from build123d import *

# Parameters (mm, degrees)
SKETCH1_W           = 69.85
SKETCH1_H           = 25.4
SKETCH1_R           = 6.35
BOSS_EXTRUDE1_DEPTH = 6.35
SKETCH3_W           = 81.28
SKETCH3_H           = 25.4
BOSS_EXTRUDE2_DEPTH = 6.35
SKETCH4_R           = 3.175
SKETCH4_R_2         = 2.2479
CUT_EXTRUDE2_DEPTH  = 118.069272335
SKETCH5_R           = 2.2479
CUT_EXTRUDE3_DEPTH  = 118.069272335


with BuildPart() as part:
    # Sketch1 → Boss-Extrude1 (new body)
    with BuildSketch(Plane(origin=(0, 0, 0), x_dir=(1, 0, 0), z_dir=(0, 1, 0))):
        Rectangle(SKETCH1_W, SKETCH1_H)
        with Locations(Location((15.875, 0, 0), (0, 0, 270))):
            Circle(SKETCH1_R, mode=Mode.SUBTRACT)
    extrude(amount=BOSS_EXTRUDE1_DEPTH)

    # Sketch3 → Boss-Extrude2 (add)
    with BuildSketch(Plane.XZ):
        with Locations((-75.565, 0)):
            Rectangle(SKETCH3_W, SKETCH3_H)
    extrude(amount=-BOSS_EXTRUDE2_DEPTH)

    # Sketch4 → Cut-Extrude2 (cut, through all)
    with BuildSketch(Plane.XZ):
        with Locations(Location((-53.55992209, 0, 0), (0, 0, 270))):
            Circle(SKETCH4_R)
        with Locations(Location((-85.725, 0, 0), (0, 0, 270))):
            Circle(SKETCH4_R_2)
        with Locations(Location((-103.5685508, 0, 0), (0, 0, 270))):
            Circle(SKETCH4_R)
    extrude(amount=-CUT_EXTRUDE2_DEPTH, mode=Mode.SUBTRACT)

    # Sketch5 → Cut-Extrude3 (cut, through all)
    with BuildSketch(Plane.XZ):
        with Locations(Location((28.1813, 0, 0), (0, 0, 270))):
            Circle(SKETCH5_R)
        with Locations(Location((3.5687, 0, 0), (0, 0, 270))):
            Circle(SKETCH5_R)
    extrude(amount=-CUT_EXTRUDE3_DEPTH, mode=Mode.SUBTRACT)


solid = part.part
CAD build for the part. Positions are in the model's coordinates, mm. Coordinates: 2 decimals unless noted, no trailing zeros. Write each loop counter-clockwise with the first axis right and the second up, starting at its lowest first coordinate (ties: lowest second). Pieces come first, ordered by that corner, then holes. Notation, with made-up numbers: (-40, -7.5) - (3, -7.5) arc R22 ccw to (3, 5.5) - close; hole circle Ø10 at (-28, 89). An arc over 180 degrees is marked (long way). Use a Markdown table: item, result. Add a question column.
Item 1: Band-saw the part on A-A, the plane z = 0. Give the cut face in (x, y) (3 decimals).
Item 2: Drill centre lines: L1, parallel to X at y = 5, z = 2.5 (3 decimals); L2, parallel to Z at x = -104, y = 1.75; L3, parallel to Z at x = -87.5, y = 4.75. Where is each one in solid material? Low to high. Write a range as from..to.
Item 3: Flat gauge pins, fed straight in: pin 1 (4 mm diameter, centred on x = 8.5, z = -2, fed in from -Y); pin 2 (2.5 mm diameter, centred on x = 28.18, z = 0, fed in from -Y). Where does each tip first touch, or does it go through?
Item 4: Band-saw the part on B-B, the plane y = 1.5. Give the cut face in (x, z) (3 decimals), and give its area (3 significant figures).
Item 5: Mould opens along X. For faces 1 (the face through (9.676, 3.131, -1.377)), 2 (the face through (34.925, 3, 0)), 3 (the face through (-50.883, 3.131, -1.707)), 4 (the face through (-42, 6.35, 0)) say: pulls with the +X half, pulls with the -X half, needs draft (parallel to the pull), parting line crosses it, or undercut.
Numbers:
| question | item | result |
|---|---|---|
| 1 | outline | (-116.205, 0) - (-106.744, 0) - (-106.744, 6.35) - (-116.205, 6.35) - close; (-100.394, 0) - (-87.973, 0) - (-87.973, 6.35) - (-100.394, 6.35) - close; (-83.477, 0) - (-56.735, 0) - (-56.735, 6.35) - (-83.477, 6.35) - close; (-50.385, 0) - (1.321, 0) - (1.321, 6.35) - (-50.385, 6.35) - close; (5.817, 0) - (9.525, 0) - (9.525, 6.35) - (5.817, 6.35) - close; (22.225, 0) - (25.933, 0) - (25.933, 6.35) - (22.225, 6.35) - close; (30.429, 0) - (34.925, 0) - (34.925, 6.35) - (30.429, 6.35) - close |
| 2 | L1 | -116.205..-105.526, -101.611..-55.517, -51.603..10.038, 21.712..34.925 |
| 2 | L2 | -12.7..-3.15, 3.15..12.7 |
| 2 | L3 | -12.7..-1.38, 1.38..12.7 |
| 3 | pin 1 | y = 0 |
| 3 | pin 2 | through |
| 4 | outline | (-116.205, -12.7) - (34.925, -12.7) - (34.925, 12.7) - (-116.205, 12.7) - close; hole circle Ø6.35 at (-103.569, 0); hole circle Ø4.496 at (-85.725, 0); hole circle Ø6.35 at (-53.56, 0); hole circle Ø4.496 at (3.569, 0); hole circle Ø12.7 at (15.875, 0); hole circle Ø4.496 at (28.181, 0) |
| 4 | area | 3,600 mm2 |
| 5 | face 1 | undercut |
| 5 | face 2 | pulls with the +X half |
| 5 | face 3 | undercut |
| 5 | face 4 | needs draft |
